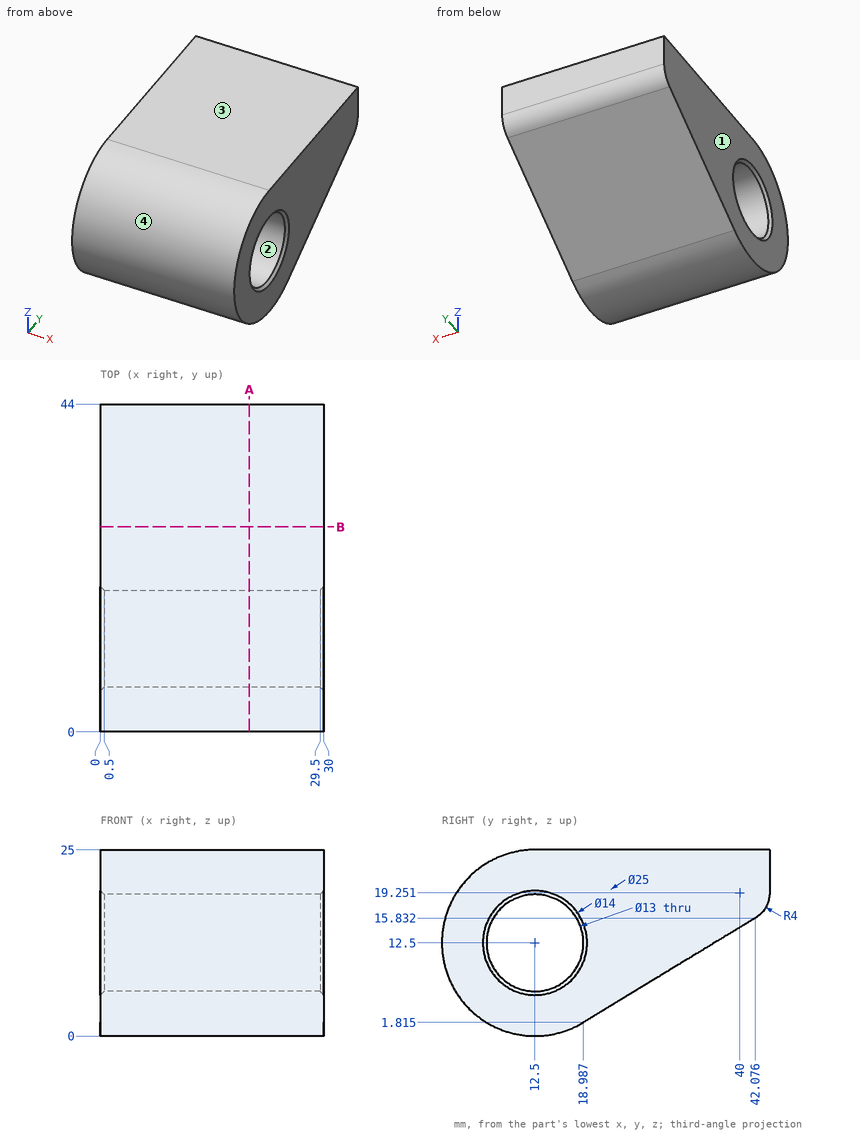
Study the drawing (mm; zero at the part's minimum x, y, z) and answer. Coordinates: 2 decimals unless noted, no trailing zeros. Write each loop counter-clockwise with the first axis right and the second up, starting at its lowest first coordinate (ties: lowest second). Pieces come first, ordered by that corner, then holes. Notation, with made-up numbers: (64.5, 37.25) -> (70.5, 37.25) arc R23 ccw to (70.5, 71.25) -> close; hole circle Ø1 at (32.5, 30.5). An arc over 180 degrees is marked (long way). Write each question's results on one line, items separated by ' | '. Start each with the question number.
1) A cutting plane is placed at B-B (y = 27.5). Determine the outline of the cut face in (x, z).
2) A cutting plane is placed at A-A (x = 20). Determine the outline of the cut face in (y, z) (1 decimal).
3) Flat-ended cylindrical pins translate along their axes: pin 1 Ø4 at (x, z) = (6, 9.5) entering from +Y; pin 2 Ø1 at (x, y) = (21.5, 30) entering from -Z. Find the tip coordinate at first contact, or state that the pin passes through.
4) For a pull along Z with two mould halves and no side action, classify the marked faces 1, 2, 3 and 4 as +Z half, -Z half, draft (parallel to the pull), parting line (faces both ways), or undercut.
5) Straight lines are drawn through the part: probe 1 along Z at (x, y) = (7, 12.5); probe 2 along Y at (x, z) = (4, 18.25) (1 decimal); probe 3 along Y at (x, z) = (25.75, 8.75) (1 decimal). For each, find the intervals that lie inside material, in ascending order.
Values follow:
1) outline: (0, 6.98) -> (30, 6.98) -> (30, 25) -> (0, 25) -> close
2) outline: (12.5, 25) arc R12.5 ccw (long way) to (19, 1.8) -> (42.1, 15.8) arc R4 ccw to (44, 19.3) -> (44, 25) -> close; hole circle Ø13 at (12.5, 12.5)
3) pin 1: y = 34.94 | pin 2: z = 8.2
4) face 1: draft | face 2: undercut | face 3: +Z half | face 4: parting line
5) probe 1: 0 to 6, 19 to 25 | probe 2: 1.4 to 9.5, 15.5 to 43.9 | probe 3: 0.6 to 7.2, 17.8 to 30.4
